Can you work these out from the model? Positions are in its coordinate system, mm. Face numbers are marked on the shaded views. A direction names the side the tool comes from. Give positions to 0.01 mm unless a question says otherwise; leave off trailing zeros. Write each loop counter-clockwise with the first axis right and the second up, starting at its lowest first coordinate (ties: lowest second). Pieces come first, ordered by that corner, then holes. Notation, with made-up numbers: (-27, 84.25) -> (19, 84.25) arc R21 ccw to (19, 123.25) -> close; hole circle Ø1 at (32.5, 62.25). An arc over 180 degrees is marked (long way). One line per item, written item: value.
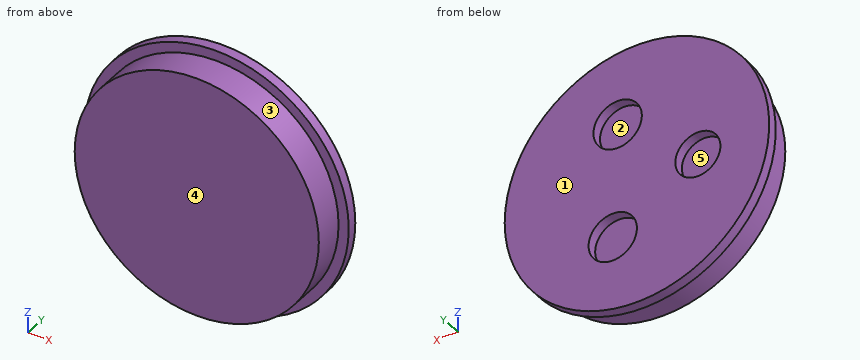
from build123d import *

# Parameters (mm, degrees)
SKETCH1_R           = 41.275
SKETCH1_R_2         = 7.05
SKETCH1_R_3         = 7.55
BOSS_EXTRUDE1_DEPTH = 3.175
SKETCH2_R           = 38.1
BOSS_EXTRUDE2_DEPTH = 9.525


with BuildPart() as part:
    # Sketch1 → Boss-Extrude1 (new body)
    with BuildSketch(Plane(origin=(0, 0, 0), x_dir=(1, 0, 0), z_dir=(0, 1, 0))):
        Circle(SKETCH1_R)
        with Locations((-19.018847828, 1.089002884)):
            Circle(SKETCH1_R_2, mode=Mode.SUBTRACT)
        with Locations((6.025718442, -18.071890251)):
            Circle(SKETCH1_R_3, mode=Mode.SUBTRACT)
        with Locations((7.550830576, 17.489638578)):
            Circle(SKETCH1_R_3, mode=Mode.SUBTRACT)
    extrude(amount=BOSS_EXTRUDE1_DEPTH)

    # Sketch2 → Boss-Extrude2 (add)
    with BuildSketch(Plane.XZ):
        Circle(SKETCH2_R)
    extrude(amount=BOSS_EXTRUDE2_DEPTH)


solid = part.part
1) If we section it at C-C (z = 21): Write out the boundary of the cut face in (x, y) (3 decimals), and give its area (3 significant figures).
Answer list:
outline: (-35.533, 0) -> (-31.79, 0) -> (-31.79, -9.525) -> (31.79, -9.525) -> (31.79, 0) -> (35.533, 0) -> (35.533, 3.175) -> (12.985, 3.175) -> (12.985, 0) -> (-0.933, 0) -> (-0.933, 3.175) -> (-35.533, 3.175) -> close
area: 787 mm^2
2) We'd pull the mould along X, two halves only. Please class the marked faces 1, 2 and 3: released by +X, released by -X, zero draft, split by the parting line, or undercut.
Answer list:
face 1: zero draft
face 2: undercut
face 3: split by the parting line
3) For the marked faces 4 and 5, which set-ups out of +Z, -Z, +X, -X, +Y, -Y let a thin tool reach every point of the face, with its end or its side?
Answer list:
face 4: +Z, -Z, +X, -X, -Y
face 5: +Y
4) Will these pins go through, and if not, where does the flat tip stop? pin 1 (7.5 mm diameter, centred on x = 10.5, z = -17, fed in from +Y); pin 2 (1.5 mm diameter, centred on y = -1.5, z = -17, fed in from +X).
Answer list:
pin 1: stops at y = 0
pin 2: stops at x = 34.46
5) If we section it at A-A (x = -16.5): Write out the boundary of the cut face in (y, z) (3 decimals), and give its area (3 significant figures).
Answer list:
outline: (-9.525, -34.342) -> (0, -34.342) -> (0, -37.834) -> (3.175, -37.834) -> (3.175, -7.674) -> (0, -7.674) -> (0, 5.496) -> (3.175, 5.496) -> (3.175, 37.834) -> (0, 37.834) -> (0, 34.342) -> (-9.525, 34.342) -> close
area: 853 mm^2
6) If we section it at D-D (z = 33.5): Write out the boundary of the cut face in (x, y) (3 decimals).
Answer list:
outline: (-24.112, 0) -> (-18.148, 0) -> (-18.148, -9.525) -> (18.148, -9.525) -> (18.148, 0) -> (24.112, 0) -> (24.112, 3.175) -> (-24.112, 3.175) -> close
7) If we section it at B-B (y = -8): Write out the boundary of the cut face in (x, z), and give its area (3 significant figures).
Answer list:
outline: circle Ø76.2 at (0, 0)
area: 4,560 mm^2
8) I need wall thicknesses on L1, parallel to X at y = 1.5, z = 21; L2, parallel to Y at x = 4, z = 22 (3 decimals); L3, parallel to X at y = 1.25, z = 2. Which ranges of each line are inside material? Lowest first, please.
Answer list:
L1: x = -35.53 to -0.93, 12.98 to 35.53
L2: y = -9.525 to 0
L3: x = -41.23 to -25.36, -12.68 to 41.23
